```python
from build123d import *

# Parameters (mm, degrees)
SKETCH_1_R               = 33.5
EXTRUDE_1_DEPTH          = 3
CUT_EXTRUDE_1_REACH      = 193.4
SKETCH_3_R               = 2
PATTERN_CIRCULAR_1_COUNT = 10
MIRROR_1_COPY_1_REACH    = 193.4
MIRROR_1_COPY_1_SKETCH_R = 2
MIRROR_1_COPY_2_REACH    = 193.4
MIRROR_1_COPY_2_SKETCH_R = 2
MIRROR_1_COPY_3_REACH    = 193.4
MIRROR_1_COPY_3_SKETCH_R = 2
MIRROR_1_COPY_4_REACH    = 193.4
MIRROR_1_COPY_4_SKETCH_R = 2
MIRROR_1_COPY_5_REACH    = 193.4
MIRROR_1_COPY_5_SKETCH_R = 2
MIRROR_1_COPY_6_REACH    = 193.4
MIRROR_1_COPY_6_SKETCH_R = 2
MIRROR_1_COPY_7_REACH    = 193.4
MIRROR_1_COPY_7_SKETCH_R = 2
MIRROR_1_COPY_8_REACH    = 193.4
MIRROR_1_COPY_8_SKETCH_R = 2
MIRROR_1_COPY_9_REACH    = 193.4
MIRROR_1_COPY_9_SKETCH_R = 2
CUT_EXTRUDE_2_REACH      = 193.4
SKETCH_4_R               = 1.5
PATTERN_LINEAR_1_COUNT   = 5
PATTERN_LINEAR_1_PITCH   = 21
CUT_EXTRUDE_3_REACH      = 193.4
SKETCH_5_R               = 1.5
PATTERN_LINEAR_2_COUNT   = 2
PATTERN_LINEAR_2_PITCH   = 50


with BuildPart() as part:
    # Sketch 1 → Extrude 1 (new body)
    with BuildSketch(Plane(origin=(0, 0, 0), x_dir=(1, 0, 0), z_dir=(0, 1, 0))):
        with BuildLine():
            Line((-150, 65), (150, 65))
            ThreePointArc((150, 65), (171.213203436, 56.213203436), (180, 35))
            Line((180, 35), (180, -35))
            ThreePointArc((180, -35), (171.213203436, -56.213203436), (150, -65))
            Line((150, -65), (-150, -65))
            ThreePointArc((-150, -65), (-171.213203436, -56.213203436), (-180, -35))
            Line((-180, -35), (-180, 35))
            ThreePointArc((-180, 35), (-171.213203436, 56.213203436), (-150, 65))
        make_face()
        with Locations(Location((105, 0, 0), (0, 0, 270))):
            Circle(SKETCH_1_R, mode=Mode.SUBTRACT)
        with Locations(Location((-105, 0, 0), (0, 0, 270))):
            Circle(SKETCH_1_R, mode=Mode.SUBTRACT)
    extrude(amount=EXTRUDE_1_DEPTH)

    # Sketch 3 → Cut-Extrude 1 (cut, up to next)
    with BuildSketch(Plane(origin=(0, 3, 0), x_dir=(1, 0, 0), z_dir=(0, 1, 0)), mode=Mode.PRIVATE) as cut_extrude_1_sk1:
        with Locations(Location((-63, 0, 0), (0, 0, 270))):
            Circle(SKETCH_3_R)
    cut_extrude_1_tool1 = extrude(cut_extrude_1_sk1.sketch, amount=-CUT_EXTRUDE_1_REACH, mode=Mode.PRIVATE) & part.part
    cut_extrude_1 = cut_extrude_1_tool1.solids().sort_by_distance((-63, 3, 0))[0]
    add(cut_extrude_1, mode=Mode.SUBTRACT)

    # Pattern Circular 1: Cut-Extrude 1 ×10 about axis
    pattern_circular_1_axis = Axis((-105, 0, 0), (0, 1, 0))
    for i in range(1, PATTERN_CIRCULAR_1_COUNT):
        add(cut_extrude_1.rotate(pattern_circular_1_axis, i * 360 / PATTERN_CIRCULAR_1_COUNT), mode=Mode.SUBTRACT)

    # Mirror 1: Cut-Extrude 1 across plane
    add(cut_extrude_1.mirror(Plane(origin=(0, 0, 0), x_dir=(0, 0, 1), z_dir=(1, 0, 0))), mode=Mode.SUBTRACT)

    # Mirror 1 copy 1 sketch → Mirror 1 copy 1 (cut, up to next)
    with BuildSketch(Plane(origin=(20.053215591, 3, -61.717451491), x_dir=(-0.8090169943749475, 0, -0.5877852522924731), z_dir=(0, 1, 0)), mode=Mode.PRIVATE) as mirror_1_copy_1_sk1:
        with Locations((-63, 0)):
            Circle(MIRROR_1_COPY_1_SKETCH_R)
    mirror_1_copy_1_tool1 = extrude(mirror_1_copy_1_sk1.sketch, amount=-MIRROR_1_COPY_1_REACH, mode=Mode.PRIVATE) & part.part
    add(mirror_1_copy_1_tool1.solids().sort_by_distance((71.021286236, 3, -24.686980596))[0], mode=Mode.SUBTRACT)

    # Mirror 1 copy 2 sketch → Mirror 1 copy 2 (cut, up to next)
    with BuildSketch(Plane(origin=(72.553215591, 3, -99.860934211), x_dir=(-0.30901699437494745, 0, -0.9510565162951535), z_dir=(0, 1, 0)), mode=Mode.PRIVATE) as mirror_1_copy_2_sk1:
        with Locations((-63, 0)):
            Circle(MIRROR_1_COPY_2_SKETCH_R)
    mirror_1_copy_2_tool1 = extrude(mirror_1_copy_2_sk1.sketch, amount=-MIRROR_1_COPY_2_REACH, mode=Mode.PRIVATE) & part.part
    add(mirror_1_copy_2_tool1.solids().sort_by_distance((92.021286236, 3, -39.944373684))[0], mode=Mode.SUBTRACT)

    # Mirror 1 copy 3 sketch → Mirror 1 copy 3 (cut, up to next)
    with BuildSketch(Plane(origin=(137.446784409, 3, -99.860934211), x_dir=(0.30901699437494734, 0, -0.9510565162951536), z_dir=(0, 1, 0)), mode=Mode.PRIVATE) as mirror_1_copy_3_sk1:
        with Locations((-63, 0)):
            Circle(MIRROR_1_COPY_3_SKETCH_R)
    mirror_1_copy_3_tool1 = extrude(mirror_1_copy_3_sk1.sketch, amount=-MIRROR_1_COPY_3_REACH, mode=Mode.PRIVATE) & part.part
    add(mirror_1_copy_3_tool1.solids().sort_by_distance((117.978713764, 3, -39.944373684))[0], mode=Mode.SUBTRACT)

    # Mirror 1 copy 4 sketch → Mirror 1 copy 4 (cut, up to next)
    with BuildSketch(Plane(origin=(189.946784409, 3, -61.717451491), x_dir=(0.8090169943749473, 0, -0.5877852522924732), z_dir=(0, 1, 0)), mode=Mode.PRIVATE) as mirror_1_copy_4_sk1:
        with Locations((-63, 0)):
            Circle(MIRROR_1_COPY_4_SKETCH_R)
    mirror_1_copy_4_tool1 = extrude(mirror_1_copy_4_sk1.sketch, amount=-MIRROR_1_COPY_4_REACH, mode=Mode.PRIVATE) & part.part
    add(mirror_1_copy_4_tool1.solids().sort_by_distance((138.978713764, 3, -24.686980596))[0], mode=Mode.SUBTRACT)

    # Mirror 1 copy 5 sketch → Mirror 1 copy 5 (cut, up to next)
    with BuildSketch(Plane(origin=(210, 3, 0), x_dir=(1, 0, 0), z_dir=(0, 1, 0)), mode=Mode.PRIVATE) as mirror_1_copy_5_sk1:
        with Locations((-63, 0)):
            Circle(MIRROR_1_COPY_5_SKETCH_R)
    mirror_1_copy_5_tool1 = extrude(mirror_1_copy_5_sk1.sketch, amount=-MIRROR_1_COPY_5_REACH, mode=Mode.PRIVATE) & part.part
    add(mirror_1_copy_5_tool1.solids().sort_by_distance((147, 3, 0))[0], mode=Mode.SUBTRACT)

    # Mirror 1 copy 6 sketch → Mirror 1 copy 6 (cut, up to next)
    with BuildSketch(Plane(origin=(189.946784409, 3, 61.717451491), x_dir=(0.8090169943749476, 0, 0.587785252292473), z_dir=(0, 1, 0)), mode=Mode.PRIVATE) as mirror_1_copy_6_sk1:
        with Locations((-63, 0)):
            Circle(MIRROR_1_COPY_6_SKETCH_R)
    mirror_1_copy_6_tool1 = extrude(mirror_1_copy_6_sk1.sketch, amount=-MIRROR_1_COPY_6_REACH, mode=Mode.PRIVATE) & part.part
    add(mirror_1_copy_6_tool1.solids().sort_by_distance((138.978713764, 3, 24.686980596))[0], mode=Mode.SUBTRACT)

    # Mirror 1 copy 7 sketch → Mirror 1 copy 7 (cut, up to next)
    with BuildSketch(Plane(origin=(137.446784409, 3, 99.860934211), x_dir=(0.30901699437494756, 0, 0.9510565162951535), z_dir=(0, 1, 0)), mode=Mode.PRIVATE) as mirror_1_copy_7_sk1:
        with Locations((-63, 0)):
            Circle(MIRROR_1_COPY_7_SKETCH_R)
    mirror_1_copy_7_tool1 = extrude(mirror_1_copy_7_sk1.sketch, amount=-MIRROR_1_COPY_7_REACH, mode=Mode.PRIVATE) & part.part
    add(mirror_1_copy_7_tool1.solids().sort_by_distance((117.978713764, 3, 39.944373684))[0], mode=Mode.SUBTRACT)

    # Mirror 1 copy 8 sketch → Mirror 1 copy 8 (cut, up to next)
    with BuildSketch(Plane(origin=(72.553215591, 3, 99.860934211), x_dir=(-0.30901699437494723, 0, 0.9510565162951536), z_dir=(0, 1, 0)), mode=Mode.PRIVATE) as mirror_1_copy_8_sk1:
        with Locations((-63, 0)):
            Circle(MIRROR_1_COPY_8_SKETCH_R)
    mirror_1_copy_8_tool1 = extrude(mirror_1_copy_8_sk1.sketch, amount=-MIRROR_1_COPY_8_REACH, mode=Mode.PRIVATE) & part.part
    add(mirror_1_copy_8_tool1.solids().sort_by_distance((92.021286236, 3, 39.944373684))[0], mode=Mode.SUBTRACT)

    # Mirror 1 copy 9 sketch → Mirror 1 copy 9 (cut, up to next)
    with BuildSketch(Plane(origin=(20.053215591, 3, 61.717451491), x_dir=(-0.8090169943749473, 0, 0.5877852522924734), z_dir=(0, 1, 0)), mode=Mode.PRIVATE) as mirror_1_copy_9_sk1:
        with Locations((-63, 0)):
            Circle(MIRROR_1_COPY_9_SKETCH_R)
    mirror_1_copy_9_tool1 = extrude(mirror_1_copy_9_sk1.sketch, amount=-MIRROR_1_COPY_9_REACH, mode=Mode.PRIVATE) & part.part
    add(mirror_1_copy_9_tool1.solids().sort_by_distance((71.021286236, 3, 24.686980596))[0], mode=Mode.SUBTRACT)

    # Sketch 4 → Cut-Extrude 2 (cut, up to next)
    with BuildSketch(Plane(origin=(0, 3, 0), x_dir=(1, 0, 0), z_dir=(0, 1, 0)), mode=Mode.PRIVATE) as cut_extrude_2_sk1:
        with Locations(Location((42, 50, 0), (0, 0, 270))):
            Circle(SKETCH_4_R)
    cut_extrude_2_tool1 = extrude(cut_extrude_2_sk1.sketch, amount=-CUT_EXTRUDE_2_REACH, mode=Mode.PRIVATE) & part.part
    cut_extrude_2 = cut_extrude_2_tool1.solids().sort_by_distance((42, 3, -50))[0]
    add(cut_extrude_2, mode=Mode.SUBTRACT)

    # Pattern Linear 1: Cut-Extrude 2 ×5
    with Locations(*[(-i * PATTERN_LINEAR_1_PITCH, 0, 0) for i in range(1, PATTERN_LINEAR_1_COUNT)]):
        add(cut_extrude_2, mode=Mode.SUBTRACT)

    # Sketch 5 → Cut-Extrude 3 (cut, up to next)
    with BuildSketch(Plane(origin=(0, 3, 0), x_dir=(1, 0, 0), z_dir=(0, 1, 0)), mode=Mode.PRIVATE) as cut_extrude_3_sk1:
        with Locations(Location((42, 0, 0), (0, 0, 270))):
            Circle(SKETCH_5_R)
    cut_extrude_3_tool1 = extrude(cut_extrude_3_sk1.sketch, amount=-CUT_EXTRUDE_3_REACH, mode=Mode.PRIVATE) & part.part
    # Sketch 5 → Cut-Extrude 3 (cut, up to next)
    with BuildSketch(Plane(origin=(0, 3, 0), x_dir=(1, 0, 0), z_dir=(0, 1, 0)), mode=Mode.PRIVATE) as cut_extrude_3_sk2:
        with Locations(Location((0, 0, 0), (0, 0, 270))):
            Circle(SKETCH_5_R)
    cut_extrude_3_tool2 = extrude(cut_extrude_3_sk2.sketch, amount=-CUT_EXTRUDE_3_REACH, mode=Mode.PRIVATE) & part.part
    # Sketch 5 → Cut-Extrude 3 (cut, up to next)
    with BuildSketch(Plane(origin=(0, 3, 0), x_dir=(1, 0, 0), z_dir=(0, 1, 0)), mode=Mode.PRIVATE) as cut_extrude_3_sk3:
        with Locations(Location((-42, 0, 0), (0, 0, 270))):
            Circle(SKETCH_5_R)
    cut_extrude_3_tool3 = extrude(cut_extrude_3_sk3.sketch, amount=-CUT_EXTRUDE_3_REACH, mode=Mode.PRIVATE) & part.part
    cut_extrude_3_1 = cut_extrude_3_tool1.solids().sort_by_distance((42, 3, 0))[0]
    add(cut_extrude_3_1, mode=Mode.SUBTRACT)
    cut_extrude_3_2 = cut_extrude_3_tool2.solids().sort_by_distance((0, 3, 0))[0]
    add(cut_extrude_3_2, mode=Mode.SUBTRACT)
    cut_extrude_3_3 = cut_extrude_3_tool3.solids().sort_by_distance((-42, 3, 0))[0]
    add(cut_extrude_3_3, mode=Mode.SUBTRACT)
    cut_extrude_3 = cut_extrude_3_1 + cut_extrude_3_2 + cut_extrude_3_3  # Cut-Extrude 3 as one shape, for the pattern or mirror that repeats it

    # Pattern Linear 2: Cut-Extrude 3 ×2
    with Locations(*[(0, 0, i * PATTERN_LINEAR_2_PITCH) for i in range(1, PATTERN_LINEAR_2_COUNT)]):
        add(cut_extrude_3, mode=Mode.SUBTRACT)


solid = part.part
```
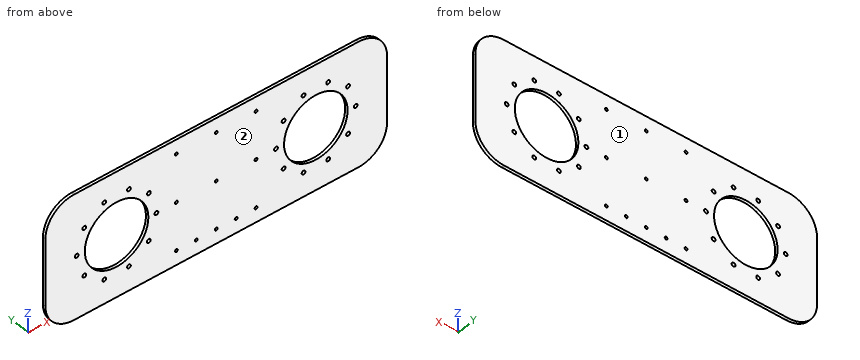
Model file for the job. Use its own axes, mm. Face numbers are marked on the shaded views. Coordinates: 2 decimals unless noted, no trailing zeros. Loops run counter-clockwise (first coordinate to the right, second up) from the corner with the lowest first, then second, coordinate; pieces in that order, holes last. Notation, with made-up numbers: M 66,64 L 119,64 A21 ccw 119,72 Z; hole C 24,75 d7. An arc over 180 degrees is marked long. Use CSV: the item, a comma, the result in double quotes. Start each with the question number.
1. Flat gauge pins, fed straight in: pin 1 (5 mm diameter, centred on x = 0, z = 0, fed in from +Y); pin 2 (3 mm diameter, centred on x = 117.98, z = 39.94, fed in from -Y). Where does each tip first touch, or does it go through?
2. Band-saw the part on A-A, the plane z = -9. List the corners of the cut face in (x, y), then the cut area to 3 significant figures.
3. Band-saw the part on C-C, the plane x = -84. List the corners of the cut face in (y, z), then the cut area to 3 significant figures.
4. Band-saw the part on B-B, the plane x = 105. List the corners of the cut face in (y, z).
5. Probe probe 1 along X at (y, z) = (2.7, -3); probe 2 along X at (y, z) = (0.65, 11); probe 3 along Z at (x, y) = (104.5, 2.3). List the from-to ranges inside material, lowest first. Write a range as [from, to].
6. Two-plate mould, pull along Y, no slides. Class the marked faces 1 and 2: pulls with the +Y half, pulls with the -Y half, needs draft (parallel to the pull), parting line crosses it, or undercut.
7. Band-saw the part on D-D, the plane z = 10. List the corners of the cut face in (x, y).
Entries:
1,pin 1,"stops at y = 3"
1,pin 2,"passes through"
2,outline,"M -180,0 L -137.27,0 L -137.27,3 L -180,3 Z; M -72.73,0 L 72.73,0 L 72.73,3 L -72.73,3 Z; M 137.27,0 L 180,0 L 180,3 L 137.27,3 Z"
2,area,"693 mm2"
3,outline,"M 0,-65 L 3,-65 L 3,-26.1 L 0,-26.1 Z; M 0,26.1 L 3,26.1 L 3,65 L 0,65 Z"
3,area,"233 mm2"
4,outline,"M 0,-65 L 3,-65 L 3,-33.5 L 0,-33.5 Z; M 0,33.5 L 3,33.5 L 3,65 L 0,65 Z"
5,probe 1,"x = [-180, -138.37], [-71.63, 71.63], [138.37, 180]"
5,probe 2,"x = [-180, -136.64], [-73.36, 73.36], [136.64, 180]"
5,probe 3,"z = [-65, -33.5], [33.5, 65]"
6,face 1,"pulls with the +Y half"
6,face 2,"pulls with the -Y half"
7,outline,"M -180,0 L -136.97,0 L -136.97,3 L -180,3 Z; M -73.03,0 L 73.03,0 L 73.03,3 L -73.03,3 Z; M 136.97,0 L 180,0 L 180,3 L 136.97,3 Z"
